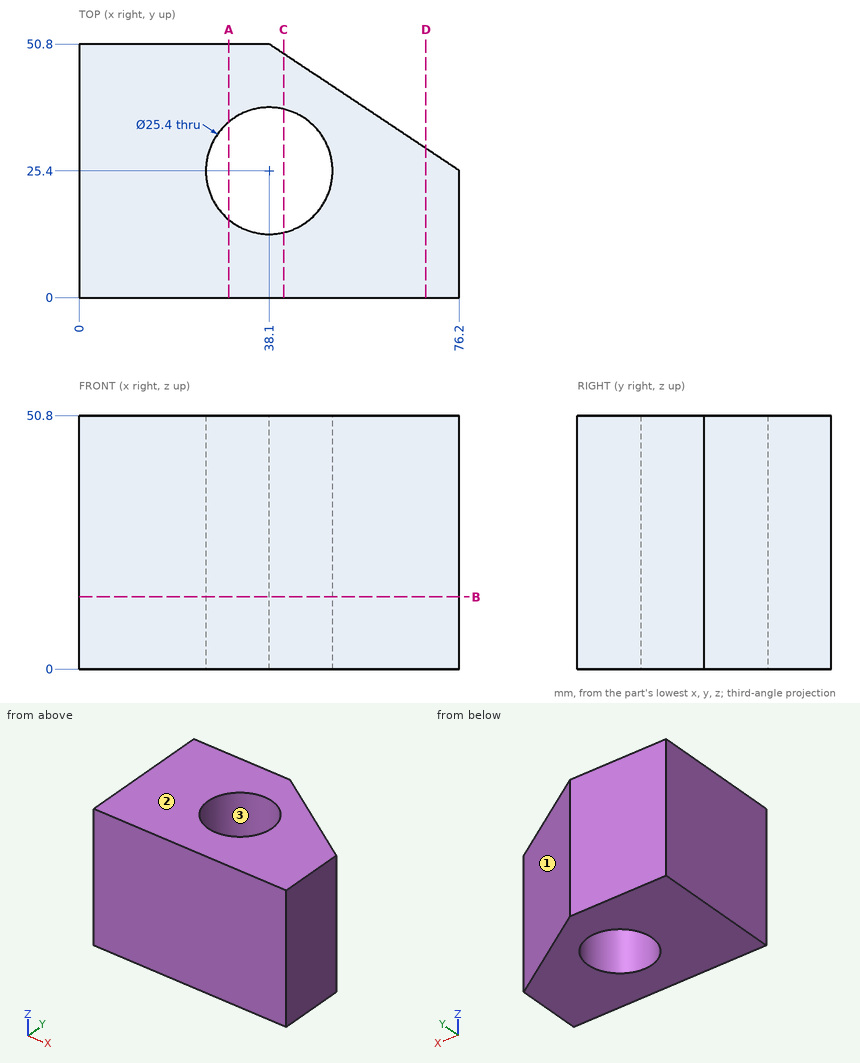
Answer from the drawing. Dimensions are ordinates in mm from the lowest x, y and z of the part. Round coordinates to 2 decimals unless told otherwise and drop trailing zeros. Write each loop counter-clockwise with the first axis right and the second up, starting at its lowest first coordinate (ties: lowest second). Pieces come first, ordered by that corner, then holes.
1. Determine the mould class of the marked faces 1, 2 and 3 for opening direction Y: pulls with the +Y half, pulls with the -Y half, needs draft (parallel to the pull), parting line crosses it, or undercut.
2. The part is cut by section D-D, the plane x = 69.5. Determine the outline of the cut face in (y, z), then the cut area to 3 significant figures.
3. Given pin 1 Ø1 at (x, z) = (51, 19) entering from +Y, flat-ended and moving along its own axis, determine where the tip first touches the part or whether it passes through.
4. The part is cut by section B-B, the plane z = 14.5. Determine the outline of the cut face in (x, y).
5. Straight lines are drawn through the part: L1, parallel to X at y = 25, z = 21; L2, parallel to Y at x = 38.1, z = 30; L3, parallel to Y at x = 36, z = 37.5. For each, find the intervals that lie inside material, in ascending order.
6. The part is cut by section C-C, the plane x = 41. Determine the outline of the cut face in (y, z), then the cut area to 3 significant figures.
7. The part is cut by section A-A, the plane x = 30. Determine the outline of the cut face in (y, z).
Values:
1. face 1: pulls with the +Y half
1. face 2: needs draft
1. face 3: undercut
2. outline: (0, 0) - (29.87, 0) - (29.87, 50.8) - (0, 50.8) - close
2. area: 1,520 mm2
3. pin 1: stops at y = 42.53
4. outline: (0, 0) - (76.2, 0) - (76.2, 25.4) - (38.1, 50.8) - (0, 50.8) - close; hole circle Ø25.4 at (38.1, 25.4)
5. L1: x = 0 to 25.41, 50.79 to 76.2
5. L2: y = 0 to 12.7, 38.1 to 50.8
5. L3: y = 0 to 12.87, 37.93 to 50.8
6. outline: (0, 0) - (13.04, 0) - (13.04, 50.8) - (0, 50.8) - close; (37.76, 0) - (48.87, 0) - (48.87, 50.8) - (37.76, 50.8) - close
6. area: 1,230 mm2
7. outline: (0, 0) - (15.62, 0) - (15.62, 50.8) - (0, 50.8) - close; (35.18, 0) - (50.8, 0) - (50.8, 50.8) - (35.18, 50.8) - close
